```python
from build123d import *

# Parameters (mm, degrees)
SKETCH1_W           = 80
SKETCH1_H           = 50
BOSS_EXTRUDE1_DEPTH = 1
SKETCH4_W           = 19.2
SKETCH4_H           = 13
SKETCH4_W_2         = 19.5
SKETCH4_H_2         = 19.5
CUT_EXTRUDE1_DEPTH  = 1
SKETCH5_R           = 2.5
BOSS_EXTRUDE2_DEPTH = 13
FILLET1_R           = 2.5
SKETCH6_W           = 21.5
SKETCH6_H           = 21.5
SKETCH6_W_2         = 19.5
SKETCH6_H_2         = 19.5
BOSS_EXTRUDE3_DEPTH = 5
SKETCH7_R           = 1.5
CUT_EXTRUDE2_DEPTH  = 10


with BuildPart() as part:
    # Sketch1 → Boss-Extrude1 (new body)
    with BuildSketch(Plane(origin=(0, 0, 0), x_dir=(0, 1, 0), z_dir=(0, 0, 1))):
        Rectangle(SKETCH1_W, SKETCH1_H)
    extrude(amount=BOSS_EXTRUDE1_DEPTH)

    # Sketch4 → Cut-Extrude1 (cut)
    with BuildSketch(Plane(origin=(0, 0, 0), x_dir=(1, 0, 0), z_dir=(0, 0, -1))):
        with Locations((0, 23.5)):
            Rectangle(SKETCH4_W, SKETCH4_H)
        with Locations((0, 5.5)):
            Rectangle(SKETCH4_W, SKETCH4_H)
        with Locations((0, -20.25)):
            Rectangle(SKETCH4_W_2, SKETCH4_H_2)
    extrude(amount=-CUT_EXTRUDE1_DEPTH, mode=Mode.SUBTRACT)

    # Sketch5 → Boss-Extrude2 (add)
    with BuildSketch(Plane(origin=(0, 0, 0), x_dir=(1, 0, 0), z_dir=(0, 0, -1))):
        with Locations(Location((0, 37.5, 0), (0, 0, 90))):
            Circle(SKETCH5_R)
        with Locations(Location((-22.5, 37.5, 0), (0, 0, 180))):
            Circle(SKETCH5_R)
        with Locations((22.5, 37.5)):
            Circle(SKETCH5_R)
        with Locations(Location((-22.5, 0, 0), (0, 0, 180))):
            Circle(SKETCH5_R)
        with Locations((22.5, 0)):
            Circle(SKETCH5_R)
        with Locations((22.5, -37.5)):
            Circle(SKETCH5_R)
        with Locations(Location((-22.5, -37.5, 0), (0, 0, 180))):
            Circle(SKETCH5_R)
        with Locations(Location((0, -37.5, 0), (0, 0, 270))):
            Circle(SKETCH5_R)
    extrude(amount=BOSS_EXTRUDE2_DEPTH)

    # Fillet1
    fillet1_edges = [part.edges().sort_by_distance(p)[0] for p in [
        (25, 40, 0.5),
        (25, -40, 0.5),
        (-25, -40, 0.5),
    ]]
    fillet(fillet1_edges, radius=FILLET1_R - 0.0001)  # a hair under: the kernel refuses the full size

    # Sketch6 → Boss-Extrude3 (add)
    with BuildSketch(Plane(origin=(0, 0, 0), x_dir=(1, 0, 0), z_dir=(0, 0, -1))):
        with Locations((0, -20.25)):
            Rectangle(SKETCH6_W, SKETCH6_H)
        with Locations((0, -20.25)):
            Rectangle(SKETCH6_W_2, SKETCH6_H_2, mode=Mode.SUBTRACT)
    extrude(amount=BOSS_EXTRUDE3_DEPTH)

    # Sketch7 → Cut-Extrude2 (cut)
    with BuildSketch(Plane(origin=(0, 0, -13), x_dir=(1, 0, 0), z_dir=(0, 0, -1))):
        with Locations(Location((-22.5, 37.5, 0), (0, 0, 180))):
            Circle(SKETCH7_R)
        with Locations(Location((0, 37.5, 0), (0, 0, 180))):
            Circle(SKETCH7_R)
        with Locations(Location((22.5, 37.5, 0), (0, 0, 180))):
            Circle(SKETCH7_R)
        with Locations(Location((-22.5, 0, 0), (0, 0, 180))):
            Circle(SKETCH7_R)
        with Locations(Location((22.5, 0, 0), (0, 0, 180))):
            Circle(SKETCH7_R)
        with Locations(Location((22.5, -37.5, 0), (0, 0, 180))):
            Circle(SKETCH7_R)
        with Locations(Location((0, -37.5, 0), (0, 0, 180))):
            Circle(SKETCH7_R)
        with Locations(Location((-22.5, -37.5, 0), (0, 0, 180))):
            Circle(SKETCH7_R)
    extrude(amount=-CUT_EXTRUDE2_DEPTH, mode=Mode.SUBTRACT)


solid = part.part
```
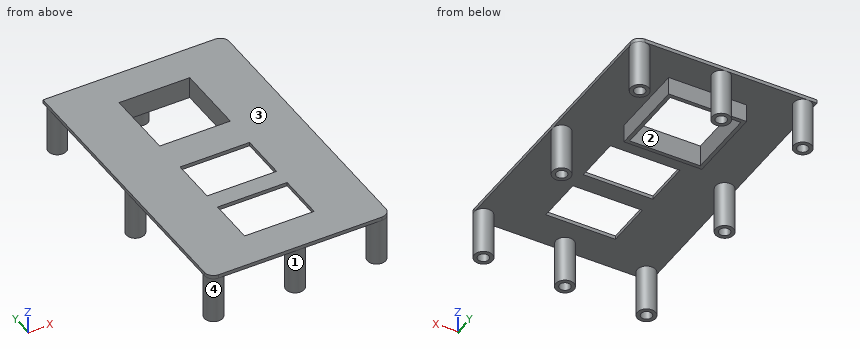
CAD build for the part. Positions are in the model's coordinates, mm. Face numbers are marked on the shaded views. A direction names the side the tool comes from. Round coordinates to 2 decimals unless told otherwise and drop trailing zeros. Loops run counter-clockwise (first coordinate to the right, second up) from the corner with the lowest first, then second, coordinate; pieces in that order, holes last. Notation, with made-up numbers: M 81,32.5 L 130,32.5 A32 cw 130,71.5 Z; hole C -19.5,65.5 d10. An arc over 180 degrees is marked long. Use a Markdown table: item, result. Add a question column.
(1) Cut at A-A (z = -7.25). State how many separate pieces and enclosed holes the cut face has, and give its area (3 significant figures).
(2) Drill centre lines: line 1 (Y direction, x = -22.5, z = -8.25); line 2 (X direction, y = 35.5, z = -9.25); line 3 (Y direction, x = -1, z = -7.5). Where is each one in solid material? Low to high.
(3) Cut at C-C (y = 16). Give the cut face in (x, z), and give its area (3 significant figures).
(4) Flat gauge pins, fed straight in: pin 1 (0.9 mm diameter, centred on x = -23, y = 0, fed in from -Z); pin 2 (2.5 mm diameter, centred on y = 25, z = -1.5, fed in from +X); pin 3 (8 mm diameter, centred on x = -13.5, y = -12, fed in from -Z); pin 4 (4 mm diameter, centred on y = -6.5, z = -2.5, fed in from +X). Where does each tip first touch, or does it go through?
(5) Pull direction X, two halves, no side cores. Call the marked faces 3 and 4: +X half, -X half, draft (parallel to the pull), parting line (faces both ways), or undercut.
(6) Which spindle directions (+Z, -Z, +X, -X, +Y, -Y) get a long thin tool onto all of the face, cutting with end or side? Do the marked faces 1 and 2. Say none if no direction does.
(7) Cut at D-D (y = -23.5). Give the cut face in (x, z).
Geometry says:
| question | item | result |
|---|---|---|
| 1 | separate pieces | 8 |
| 1 | enclosed holes | 8 |
| 1 | area | 101 mm² |
| 2 | line 1 | y = -40 to -39, -36 to -35, -2.5 to -1.5, 1.5 to 2.5, 35 to 36, 39 to 40 |
| 2 | line 2 | x = -24 to -21, -1.5 to 1.5, 21 to 24 |
| 2 | line 3 | y = -39.79 to -38.62, -36.38 to -35.21, 35.21 to 36.38, 38.62 to 39.79 |
| 3 | outline | M -25,0 L -10.75,0 L -10.75,-5 L -9.75,-5 L -9.75,1 L -25,1 Z; M 9.75,-5 L 10.75,-5 L 10.75,0 L 25,0 L 25,1 L 9.75,1 Z |
| 3 | area | 40.5 mm² |
| 4 | pin 1 | stops at z = -3 |
| 4 | pin 2 | stops at x = 10.75 |
| 4 | pin 3 | stops at z = 0 |
| 4 | pin 4 | passes through |
| 5 | face 3 | draft |
| 5 | face 4 | undercut |
| 6 | face 1 | -Z |
| 6 | face 2 | +Z, -Z |
| 7 | outline | M -25,0 L -9.6,0 L -9.6,1 L -25,1 Z; M 9.6,0 L 25,0 L 25,1 L 9.6,1 Z |
